```python
from build123d import *

# Parameters (mm, degrees)
CUT_EXTRUDE2_DEPTH = 8.62
CUT_EXTRUDE3_DEPTH = 8.62
CHAMFER1_SIZE      = 1.016
CHAMFER2_SIZE      = 0.508


with BuildPart() as part:
    # Sketch1 → Revolve1 (revolve)
    with BuildSketch(Plane.XY):
        Polygon((0, 0), (0, -7.62), (25.0698, -7.62), (25.0698, -3.6576), (30.0228, -3.6576), (30.0228, 0), align=None)
    revolve(axis=Axis((0, -1000, 0), (0, 1, 0)))

    # Sketch3 → Cut-Extrude2 (cut, through all)
    with BuildSketch(Plane(origin=(0, 0, 0), x_dir=(1, 0, 0), z_dir=(0, 1, 0))):
        with BuildLine():
            Line((-0.635, 9.525), (0.635, 9.525))
            Line((0.635, 9.525), (0.635, -30.016083936))
            ThreePointArc((0.635, -30.016083936), (0, -30.0228), (-0.635, -30.016083936))
            Line((-0.635, -30.016083936), (-0.635, 9.525))
        make_face()
    extrude(amount=-CUT_EXTRUDE2_DEPTH, mode=Mode.SUBTRACT)

    # Sketch5 → Cut-Extrude3 (cut, through all)
    with BuildSketch(Plane(origin=(0, 0, 0), x_dir=(1, 0, 0), z_dir=(0, 1, 0))):
        with BuildLine():
            Line((-1.9558, 29.959028125), (-1.9558, 27.9908))
            ThreePointArc((-1.9558, 27.9908), (0, 26.035), (1.9558, 27.9908))
            Line((1.9558, 27.9908), (1.9558, 29.959028125))
            ThreePointArc((1.9558, 29.959028125), (0, 30.0228), (-1.9558, 29.959028125))
        make_face()
    extrude(amount=-CUT_EXTRUDE3_DEPTH, mode=Mode.SUBTRACT)

    # Chamfer1
    chamfer1_edges = [part.edges().sort_by_distance(p)[0] for p in [
        (-30.015522282, -3.6576, 0.661015886),
        (-17.501079239, -7.62, -17.950128064),
        (30.015522282, -3.6576, 0.661015886),
    ]]
    chamfer(chamfer1_edges, length=CHAMFER1_SIZE)

    # Chamfer2
    chamfer2_edges = [part.edges().sort_by_distance(p)[0] for p in [
        (-30.015522282, 0, 0.661015886),
        (-0.635, 0, 10.245541968),
        (0.635, 0, 10.245541968),
        (0, 0, -9.525),
        (30.015522282, 0, 0.661015886),
        (-1.9558, 0, -28.974914063),
        (0, 0, -26.035),
        (1.9558, 0, -28.974914063),
    ]]
    chamfer(chamfer2_edges, length=CHAMFER2_SIZE)


solid = part.part
```
Design review of the part built by this model. Coordinates are the model's own, in mm. A direction names the side the tool comes from. Give positions to 0.01 mm unless a question says otherwise; leave off trailing zeros. Write each loop counter-clockwise with the first axis right and the second up, starting at its lowest first coordinate (ties: lowest second). Pieces come first, ordered by that corner, then holes. Notation, with made-up numbers: (26, 49) - (70, 49) arc R23 ccw to (70, 78) - close; hole circle Ø1 at (42, 9.25). An arc over 180 degrees is marked (long way). Return JSON: item names as keys, results as strings. Group by question number.
(1) To check wall thickness, follow probe 1 along X at (y, z) = (-3, -3) (3 decimals); probe 2 along Y at (x, z) = (24, 15); probe 3 along X at (y, z) = (-1, -7) (3 decimals). State the ranges of each line that lie inside material, in increasing order.
(2) We need section A-A, the plane y = -5.25. Give the boundary of the cut face in (x, z) (3 decimals), then the cut area to 3 significant figures.
(3) Machinability: for faces 1 (the flat face through (-1.956, -2, -29)), 2 (the flat face through (-0.635, -4, 11)), 3 (the conical face through (-0.05, -0.37, -25.9)), which of the approach directions +Z, -Z, +X, -X, +Y, -Y give a long, thin tool a straight path to every point of the face, cutting with its end or side? Answer none if there is none.
(4) Insertion check: pin 1 (1.4 mm diameter, centred on x = -0.5, y = -5.5, fed in from +Z); pin 2 (4 mm diameter, centred on x = 10.5, y = -1.5, fed in from +Z); pin 3 (1 mm diameter, centred on x = 21, z = -20.5, fed in from -Y). Each pin has a flat end and moves straight along its axis. Give the tip position at first contact, or say it passes through.
(5) Mouldability with a two-part tool opening along X and no side actions: class faces 4 (the flat face through (1.956, -2, -29)), 5 (the conical face through (-29.659, -0.145, 0.019)), 6 (the flat face through (13, -3.658, -22)) as +X half, -X half, draft (parallel to the pull), parting line (faces both ways), or undercut.
Reported:
{
 "1": {"probe 1": "x = -29.512 to -0.635, 0.635 to 29.512", "probe 2": "y = -3.66 to 0", "probe 3": "x = -29.195 to -0.635, 0.635 to 29.195"},
 "2": {"outline": "(-0.635, -9.525) - (-0.635, 25.062) arc R25.07 ccw (long way) to (0.635, 25.062) - (0.635, -9.525) - close", "area": "1,930 mm2"},
 "3": {"face 1": "-Z, +Y, -Y", "face 2": "+Z, +Y, -Y", "face 3": "-Z, +Y"},
 "4": {"pin 1": "stops at z = 25.06", "pin 2": "stops at z = 28.79", "pin 3": "stops at y = -3.66"},
 "5": {"face 4": "undercut", "face 5": "-X half", "face 6": "draft"}
}
